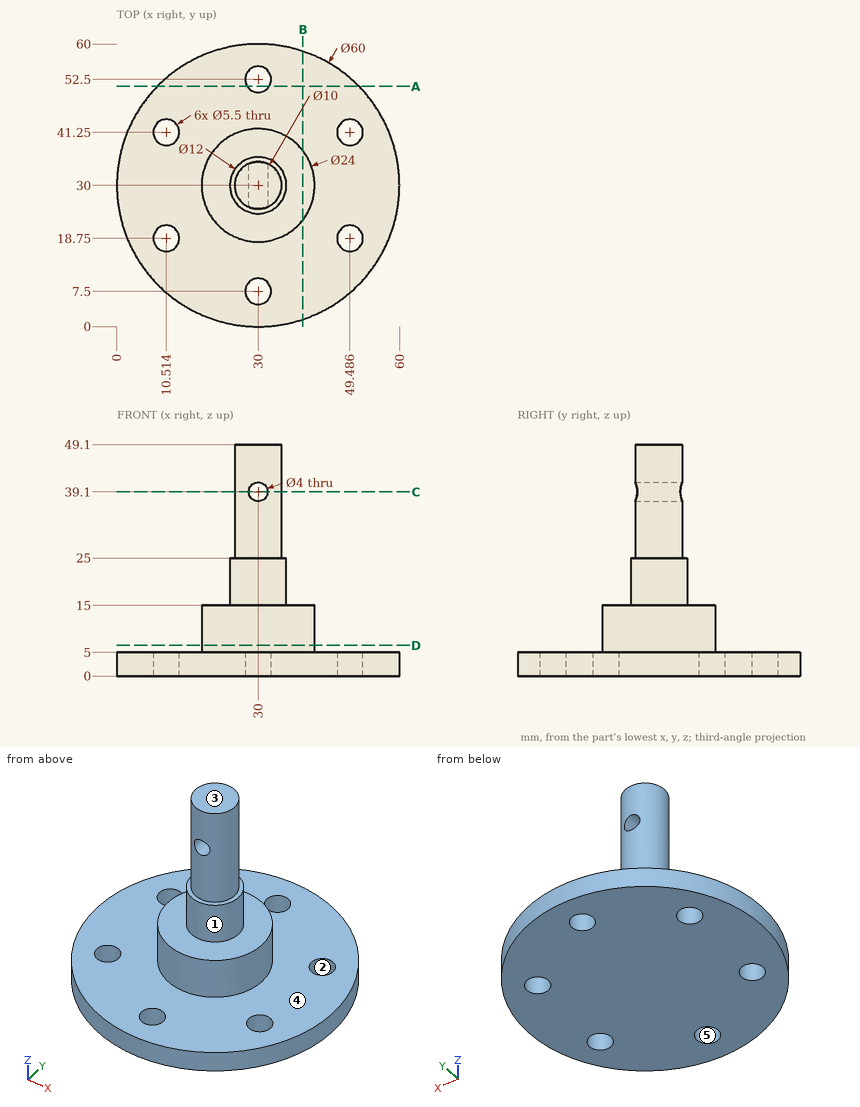
Job drawing, mm, ordinate dimensions from the low corner. One solid piece. A direction names the side the tool comes from. Give positions to 0.01 mm unless a question says otherwise; leave off trailing zeros. Write each loop counter-clockwise with the first axis right and the second up, starting at its lowest first coordinate (ties: lowest second). Pieces come first, ordered by that corner, then holes. Notation, with made-up numbers: M 60.25,56 L 90.25,56 A22 ccw 90.25,63 Z; hole C -37.5,-7.75 d2. An arc over 180 degrees is marked long. One line per item, written item: value. Start each with the question number.
Q1. Saw through at A-A, the plane y = 51. Write the cut outline in (x, z) (1 decimal), plus the area to 3 significant figures.
Q2. Two-plate mould, pull along Y, no slides. Class the marked faces 1, 2 and 3: +Y half, -Y half, draft (parallel to the pull), parting line (faces both ways), or undercut.
Q3. Saw through at B-B, the plane x = 39.5. Write the cut outline in (y, z).
Q4. Saw through at C-C, the plane z = 39.1. Write the cut outline in (x, y).
Q5. 3-axis set-ups, long thin cutter, end or side, ignore diameter. For the marked faces 4 and 5: which of +Z, -Z, +X, -X, +Y, -Y reach the whole face in a straight line?
Q6. Saw through at D-D, the plane z = 6.5. Write the cut outline in (x, y), plus the area to 3 significant figures.
Q7. Drop flat-ended pins along their axis: pin 1 Ø2.5 at (x, z) = (30, 39.1) entering from +Y; pin 2 Ø3 at (y, z) = (32.5, 23) entering from +X; pin 3 Ø12 at (y, z) = (29.5, 23.5) entering from -X; pin 4 Ø12 at (x, y) = (13.5, 42.5) entering from +Z. Give the stop position or say it passes through.
Q8. Probe probe 1 along Y at (x, z) = (30, 2.25); probe 2 along Z at (x, y) = (30, 28); probe 3 along Y at (x, z) = (29, 3). List the from-to ranges inside material, lowest first. Write a range as [from, to].
Output values:
1. outline: M 8.6,0 L 27.7,0 L 27.7,5 L 8.6,5 Z; M 32.3,0 L 51.4,0 L 51.4,5 L 32.3,5 Z
1. area: 191 mm²
2. face 1: parting line
2. face 2: undercut
2. face 3: draft
3. outline: M 1.54,0 L 58.46,0 L 58.46,5 L 37.33,5 L 37.33,15 L 22.67,15 L 22.67,5 L 1.54,5 Z
4. outline: M 28,25.42 L 28,34.58 A5 ccw Z; M 32,25.42 A5 ccw 32,34.58 Z
5. face 4: +Z
5. face 5: +Z, -Z
6. outline: C 30,30 d24
6. area: 452 mm²
7. pin 1: passes through
7. pin 2: stops at x = 35.92
7. pin 3: stops at x = 24
7. pin 4: stops at z = 5
8. probe 1: y = [0, 4.75], [10.25, 49.75], [55.25, 60]
8. probe 2: z = [0, 37.1], [41.1, 49.1]
8. probe 3: y = [0.02, 4.94], [10.06, 49.94], [55.06, 59.98]
